Can you work these out from the model? Positions are in its coordinate system, mm. A direction names the side the tool comes from. Coordinates: 2 decimals unless noted, no trailing zeros. Loops run counter-clockwise (first coordinate to the right, second up) from the corner with the lowest first, then second, coordinate; pieces in that order, holes last. Notation, with made-up numbers: (-12, 69) -> (30, 69) arc R10 ccw to (30, 83) -> close; hole circle Ø11 at (41.25, -27.75). An arc over 180 degrees is marked (long way). Put each result on its own line as item: value. Start each with the question number.
Item 1: If we section it at C-C on x = 38: Please give me the cut outline in (y, z).
Item 2: If we section it at D-D on z = -85: Please give me the cut outline in (x, y), plus the area to 3 significant figures.
Item 3: If we section it at A-A on z = -99: Please give me the cut outline in (x, y).
Item 4: We'd pull the mould along X, two halves only. Please class faces 5 (the flat face through (-14.61, 0.07, -82.85)), 6 (the flat face through (49.53, -0.07, -95.99)), 7 (the flat face through (69.633, -0.07, -61.711)): pulls with the +X half, pulls with the -X half, needs draft (parallel to the pull), parting line crosses it, or undercut.
Item 5: Please list where these lines run through material, in increasing order: L1, parallel to Z at x = 56.5, y = -2.5; L2, parallel to Z at x = -1.5, y = 1; L3, parallel to Z at x = 59, y = -1.75. Write a range as from..to.
Item 6: Will these pins go through, and if not, where does the flat tip stop? P1, Ø5, axis at y = 4, z = -108, coming from the -X side; P2, Ø1.5, axis at y = 0.5, z = -112, coming from the -X side; P3, Ø1, axis at x = 54.5, z = -103, coming from the +Y side; P4, Ø6, axis at x = 28.5, y = 4, coming from the -Z side.
Item 7: If we section it at B-B on x = 23: Please give me the cut outline in (y, z).
Item 8: For faces 1 (the flat face through (64.64, 0.07, -54.24)), 2 (the flat face through (92.72, -0.07, -81.18)), 3 (the flat face through (-13.604, -0.07, -92.045)), 4 (the flat face through (31.262, -0.07, -85.462)), which set-ups out of +Z, -Z, +X, -X, +Y, -Y let a thin tool reach every point of the face, with its end or its side?
```python
from build123d import *

# Parameters (mm, degrees)
BOSS_EXTRUDE1_START       = -5
BOSS_EXTRUDE1_OUTLINE_R   = 125
BOSS_EXTRUDE1_OUTLINE_R_2 = 2.1
BOSS_EXTRUDE1_OUTLINE_W   = 21
BOSS_EXTRUDE1_OUTLINE_H   = 31
BOSS_EXTRUDE1_OUTLINE_W_2 = 30.2
BOSS_EXTRUDE1_OUTLINE_H_2 = 10.2
BOSS_EXTRUDE1_OUTLINE_R_3 = 75.5
BOSS_EXTRUDE1_DEPTH       = 10
SKETCH4_OUTSIDE_W         = 322.738
SKETCH4_OUTSIDE_H         = 322.738
CUT_EXTRUDE1_DEPTH        = 10


# Read off the part's stored shape, not the designer's step: Boss-Extrude1
with BuildPart() as part:
    # Boss-Extrude1 outline → Boss-Extrude1 (new body)
    with BuildSketch(Plane(origin=(0, 0, 0), x_dir=(1, 0, 0), z_dir=(0, 1, 0)).offset(BOSS_EXTRUDE1_START)):
        Circle(BOSS_EXTRUDE1_OUTLINE_R)
        Polygon((-86.463555034, -86.708152159), (-66.537139134, -62.960774422), (-50.450205829, -76.459314226), (-70.376621729, -100.206691962), align=None, mode=Mode.SUBTRACT)
        Polygon((-91.105361481, -83.104052392), (-97.661795099, -75.290399072), (-74.527252917, -55.87821326), (-67.970819298, -63.69186658), align=None, mode=Mode.SUBTRACT)
        Polygon((-51.593230004, -111.051288231), (-40.990605561, -81.920816987), (-21.257060524, -89.103239996), (-31.859684967, -118.233711241), align=None, mode=Mode.SUBTRACT)
        Polygon((-16.372500708, -122.222795071), (-26.417539789, -120.451583659), (-21.173364823, -90.710389518), (-11.128325743, -92.48160093), align=None, mode=Mode.SUBTRACT)
        Polygon((-57.187775987, -109.252133582), (-66.021235106, -104.152133582), (-50.921235106, -77.998166387), (-42.087775987, -83.098166387), align=None, mode=Mode.SUBTRACT)
        Polygon((-114.034295807, -46.932395999), (-117.522901269, -37.347531267), (-89.144184122, -27.018522939), (-85.65557866, -36.603387671), align=None, mode=Mode.SUBTRACT)
        Polygon((-110.905099262, -51.90673326), (-84.058311744, -36.40673326), (-73.558311744, -54.59326674), (-100.405099262, -70.09326674), align=None, mode=Mode.SUBTRACT)
        Polygon((-121.969851733, -10.844596269), (-91.44081139, -5.461502761), (-87.794199659, -26.142465574), (-118.323240002, -31.525559082), align=None, mode=Mode.SUBTRACT)
        with Locations((-81.298478633, -10.703147762)):
            Circle(BOSS_EXTRUDE1_OUTLINE_R_2, mode=Mode.SUBTRACT)
        with Locations((0, -106.5)):
            Rectangle(BOSS_EXTRUDE1_OUTLINE_W, BOSS_EXTRUDE1_OUTLINE_H, mode=Mode.SUBTRACT)
        Polygon((26.417539789, -120.451583659), (16.372500708, -122.222795071), (11.128325743, -92.48160093), (21.173364823, -90.710389518), align=None, mode=Mode.SUBTRACT)
        Polygon((31.859684968, -118.233711241), (21.257060524, -89.103239996), (40.990605561, -81.920816987), (51.593230004, -111.051288231), align=None, mode=Mode.SUBTRACT)
        with Locations((10.703147762, -81.298478633)):
            Circle(BOSS_EXTRUDE1_OUTLINE_R_2, mode=Mode.SUBTRACT)
        Polygon((66.021235106, -104.152133582), (57.187775987, -109.252133582), (42.087775987, -83.098166387), (50.921235106, -77.998166387), align=None, mode=Mode.SUBTRACT)
        Polygon((70.376621729, -100.206691962), (50.450205829, -76.459314226), (66.537139134, -62.960774422), (86.463555035, -86.708152159), align=None, mode=Mode.SUBTRACT)
        Polygon((97.661795099, -75.290399072), (91.105361481, -83.104052392), (67.970819298, -63.69186658), (74.527252917, -55.87821326), align=None, mode=Mode.SUBTRACT)
        Polygon((100.405099262, -70.09326674), (73.558311744, -54.59326674), (84.058311744, -36.40673326), (110.905099262, -51.90673326), align=None, mode=Mode.SUBTRACT)
        Polygon((117.522901269, -37.347531267), (114.034295807, -46.932395999), (85.65557866, -36.603387671), (89.144184122, -27.018522939), align=None, mode=Mode.SUBTRACT)
        Polygon((118.323240002, -31.525559082), (87.794199659, -26.142465574), (91.44081139, -5.461502761), (121.969851733, -10.844596269), align=None, mode=Mode.SUBTRACT)
        with Locations((-108.109011093, 0)):
            Rectangle(BOSS_EXTRUDE1_OUTLINE_W_2, BOSS_EXTRUDE1_OUTLINE_H_2, mode=Mode.SUBTRACT)
        Polygon((-118.323240002, 31.525559082), (-87.794199659, 26.142465574), (-91.44081139, 5.461502761), (-121.969851733, 10.844596269), align=None, mode=Mode.SUBTRACT)
        Polygon((-117.522901269, 37.347531267), (-114.034295807, 46.932395999), (-85.65557866, 36.603387671), (-89.144184122, 27.018522939), align=None, mode=Mode.SUBTRACT)
        Polygon((-100.405099262, 70.09326674), (-73.558311744, 54.59326674), (-84.058311744, 36.40673326), (-110.905099262, 51.90673326), align=None, mode=Mode.SUBTRACT)
        Polygon((-97.661795099, 75.290399072), (-91.105361481, 83.104052392), (-67.970819298, 63.69186658), (-74.527252917, 55.87821326), align=None, mode=Mode.SUBTRACT)
        Polygon((-70.376621729, 100.206691962), (-50.450205829, 76.459314226), (-66.537139134, 62.960774422), (-86.463555035, 86.708152159), align=None, mode=Mode.SUBTRACT)
        Polygon((-66.021235106, 104.152133582), (-57.187775987, 109.252133582), (-42.087775987, 83.098166387), (-50.921235106, 77.998166387), align=None, mode=Mode.SUBTRACT)
        with Locations((-10.703147762, 81.298478633)):
            Circle(BOSS_EXTRUDE1_OUTLINE_R_2, mode=Mode.SUBTRACT)
        Polygon((-31.859684967, 118.233711241), (-21.257060524, 89.103239996), (-40.990605561, 81.920816987), (-51.593230004, 111.051288231), align=None, mode=Mode.SUBTRACT)
        Polygon((-26.417539789, 120.451583659), (-16.372500708, 122.222795071), (-11.128325743, 92.48160093), (-21.173364823, 90.710389518), align=None, mode=Mode.SUBTRACT)
        Circle(BOSS_EXTRUDE1_OUTLINE_R_3, mode=Mode.SUBTRACT)
        with Locations((81.298478633, 10.703147762)):
            Circle(BOSS_EXTRUDE1_OUTLINE_R_2, mode=Mode.SUBTRACT)
        with Locations((108.109011093, 0)):
            Rectangle(BOSS_EXTRUDE1_OUTLINE_W_2, BOSS_EXTRUDE1_OUTLINE_H_2, mode=Mode.SUBTRACT)
        Polygon((121.969851733, 10.844596269), (91.44081139, 5.461502761), (87.794199659, 26.142465574), (118.323240002, 31.525559082), align=None, mode=Mode.SUBTRACT)
        Polygon((110.905099262, 51.90673326), (84.058311744, 36.40673326), (73.558311744, 54.59326674), (100.405099262, 70.09326674), align=None, mode=Mode.SUBTRACT)
        Polygon((114.034295807, 46.932395999), (117.522901269, 37.347531267), (89.144184122, 27.018522939), (85.65557866, 36.603387671), align=None, mode=Mode.SUBTRACT)
        Polygon((57.187775987, 109.252133582), (66.021235106, 104.152133582), (50.921235106, 77.998166387), (42.087775987, 83.098166387), align=None, mode=Mode.SUBTRACT)
        with Locations((0, 106.5)):
            Rectangle(BOSS_EXTRUDE1_OUTLINE_W, BOSS_EXTRUDE1_OUTLINE_H, mode=Mode.SUBTRACT)
        Polygon((16.372500708, 122.222795071), (26.417539789, 120.451583659), (21.173364823, 90.710389518), (11.128325743, 92.48160093), align=None, mode=Mode.SUBTRACT)
        Polygon((51.593230004, 111.051288231), (40.990605561, 81.920816987), (21.257060524, 89.103239996), (31.859684967, 118.233711241), align=None, mode=Mode.SUBTRACT)
        Polygon((91.105361481, 83.104052392), (97.661795099, 75.290399072), (74.527252917, 55.87821326), (67.970819298, 63.69186658), align=None, mode=Mode.SUBTRACT)
        Polygon((86.463555035, 86.708152159), (66.537139134, 62.960774422), (50.450205829, 76.459314226), (70.376621729, 100.206691962), align=None, mode=Mode.SUBTRACT)
    extrude(amount=BOSS_EXTRUDE1_DEPTH)

    # Sketch4 outside → Cut-Extrude1 (cut)
    with BuildSketch(Plane(origin=(0, 5, 0), x_dir=(1, 0, 0), z_dir=(0, 1, 0))):
        Rectangle(SKETCH4_OUTSIDE_W, SKETCH4_OUTSIDE_H)
        with BuildLine():
            Line((-10.697510124, 60.668594683), (-21.395020248, 121.337189365))
            Line((-21.395020248, 121.337189365), (-23.360523909, 132.484114544))
            ThreePointArc((-23.360523909, 132.484114544), (45.824573947, 126.527015659), (101.778053823, 85.401927425))
            Line((101.778053823, 85.401927425), (94.38357829, 79.197225732))
            Line((94.38357829, 79.197225732), (51.307753621, 43.05231714))
            ThreePointArc((51.307753621, 43.05231714), (21.817456639, 57.183528482), (-10.697510124, 60.668594683))
        make_face(mode=Mode.SUBTRACT)
    extrude(amount=-CUT_EXTRUDE1_DEPTH, mode=Mode.SUBTRACT)


solid = part.part
```
Solutions:
1. outline: (-5, -119.08) -> (5, -119.08) -> (5, -116) -> (-5, -116) -> close; (-5, -83.01) -> (5, -83.01) -> (5, -65.24) -> (-5, -65.24) -> close
2. outline: (-14.99, -5) -> (32.53, -5) -> (32.53, 5) -> (-14.99, 5) -> close; (42.11, -5) -> (43.19, -5) -> (43.19, 5) -> (42.11, 5) -> close; (54.96, -5) -> (57.62, -5) -> (57.62, 5) -> (54.96, 5) -> close; (85.03, -5) -> (91.65, -5) -> (91.65, 5) -> (85.03, 5) -> close
2. area: 579 mm^2
3. outline: (-12.28, -5) -> (-10.5, -5) -> (-10.5, 5) -> (-12.28, 5) -> close; (10.5, -5) -> (12.28, -5) -> (12.28, 5) -> (10.5, 5) -> close; (22.64, -5) -> (24.86, -5) -> (24.86, 5) -> (22.64, 5) -> close; (47.21, -5) -> (51.27, -5) -> (51.27, 5) -> (47.21, 5) -> close; (63.05, -5) -> (69.36, -5) -> (69.36, 5) -> (63.05, 5) -> close; (71.81, -5) -> (76.32, -5) -> (76.32, 5) -> (71.81, 5) -> close
4. face 5: pulls with the -X half
4. face 6: undercut
4. face 7: pulls with the +X half
5. L1: -111.5..-108.06, -87.66..-83.67, -71.38..-50.08
5. L2: -124.99..-122, -91..-75.49
5. L3: -110.2..-108.21, -91.99..-86.65, -69.29..-49.51
6. P1: x = -14.31
6. P2: x = -14.7
6. P3: through
6. P4: z = -122.37
7. outline: (-5, -122.87) -> (5, -122.87) -> (5, -121.05) -> (-5, -121.05) -> close; (-5, -101.07) -> (5, -101.07) -> (5, -93.89) -> (-5, -93.89) -> close; (-5, -88.47) -> (5, -88.47) -> (5, -71.91) -> (-5, -71.91) -> close
8. face 1: +Z, +X, +Y, -Y
8. face 2: +Z, +Y, -Y
8. face 3: -X, +Y, -Y
8. face 4: +Y, -Y
